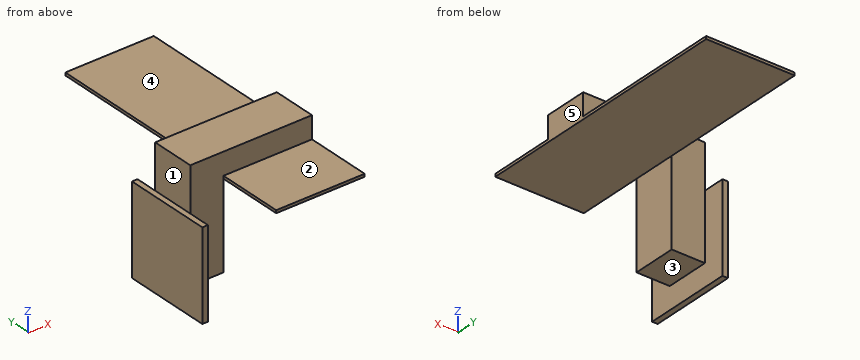
from build123d import *

# Parameters (mm, degrees)
F0_W     = 101.6
F0_H     = 304.8
F1_DEPTH = 3.175
F2_W     = 38.1
F2_H     = 50.8
F2_W_2   = 101.6
F3_DEPTH = 25.4
F4_DEPTH = 101.6
F6_DEPTH = 6.35


# Not quite as in the source:
# - the program builds the solid bodies; features that only make, move or delete a surface that nothing else refers to are left out


with BuildPart() as f1:
    # F0 (on Top) → F1 (new body)
    with BuildSketch(Plane.XY):
        with Locations((17.6723517966, 8.8070686907)):
            Rectangle(F0_W, F0_H)
    extrude(amount=F1_DEPTH)

    # F2 (on face) → F3 (join)
    with BuildSketch(Plane.XY.offset(3.175)):
        with Locations((-52.1776482034, -41.9929313093)):
            Rectangle(F2_W, F2_H)
        with Locations((17.6723517966, -41.9929313093)):
            Rectangle(F2_W_2, F2_H)
    extrude(amount=F3_DEPTH)

    # F4 (add): a face of the model
    f4_faces = [f1.faces().sort_by_distance(p)[0] for p in [
        (-52.1776482034, -41.9929313093, 3.175),
    ]]
    extrude(f4_faces, amount=F4_DEPTH)

    # F5 (on face) → F6 (join)
    with BuildSketch(Plane(origin=(-71.2276482034, 0, 0), x_dir=(0, -1, 0), z_dir=(-1, 0, 0))):
        Polygon((92.7929313093, -123.825), (92.7929313093, -22.225), (67.3929313093, -22.225), (67.3929313093, -98.425), (41.9929313093, -98.425), (16.5929313093, -98.425), (16.5929313093, -22.225), (-8.8070686907, -22.225), (-8.8070686907, -123.825), align=None)
        Polygon((67.3929313093, -98.425), (67.3929313093, -22.225), (16.5929313093, -22.225), (16.5929313093, -98.425), (41.9929313093, -98.425), align=None)
    extrude(amount=F6_DEPTH)


solid = f1.part
Geometry: final body of the model. Coordinates: model frame, mm. Face numbers are marked on the shaded views. A direction names the side the tool comes from. Give positions to 0.01 mm unless a question says otherwise; leave off trailing zeros. Loops run counter-clockwise (first coordinate to the right, second up) from the corner with the lowest first, then second, coordinate; pieces in that order, holes last. Notation, with made-up numbers: (6.5, 86) -> (52.5, 86) arc R34 cw to (52.5, 118) -> close; hole circle Ø1 at (59.25, -17.75). An arc over 180 degrees is marked (long way). Put each result on its own line as item: value.
1. Cut plane A-A (y = -84). Return the cut outline in (x, z) (3 decimals), plus the area to 3 significant figures.
Taken from the geometry:
outline: (-77.578, -123.825) -> (-71.228, -123.825) -> (-71.228, -22.225) -> (-77.578, -22.225) -> close; (-33.128, 0) -> (68.472, 0) -> (68.472, 3.175) -> (-33.128, 3.175) -> close
area: 968 mm2
2. Cut plane D-D (y = -32.5). Return the cut outline in (x, z) (3 decimals).
Taken from the geometry:
outline: (-77.578, -123.825) -> (-71.228, -123.825) -> (-71.228, -98.425) -> (-33.128, -98.425) -> (-33.128, 0) -> (68.472, 0) -> (68.472, 28.575) -> (-71.228, 28.575) -> (-71.228, -22.225) -> (-77.578, -22.225) -> close
3. Pin query (flat end, axial travel): P1, Ø1.6, axis at y = 97.5, z = 2, coming from the -X side; P2, Ø11.5, axis at x = -53.5, y = -50, coming from the -Z side (3 decimals); P3, Ø2, axis at x = 46, y = -104, coming from the -Z side. Return the tip coordinate at first contact, or that it passes through.
Taken from the geometry:
P1: stops at x = -33.13
P2: stops at z = -98.425
P3: stops at z = 0
4. Ray query, line 1 along Z through (x, y) = (-22, -116.5) (3 decimals); line 2 along X through (y, z) = (-23.5, -114.5); line 3 along X through (y, z) = (-57.5, -22). Return the intervals inside material, ascending. Write a range as [from, to].
Taken from the geometry:
line 1: z = [0, 3.175]
line 2: x = [-77.58, -71.23]
line 3: x = [-71.23, -33.13]
5. Set-up query: the marked faces 1, 2, 3, 4 and 5. Return all of +Z, -Z, +X, -X, +Y, -Y with unobstructed straight access to the full face (end or side cutting, diameter ignored); none if empty.
Taken from the geometry:
face 1: +Z, -X, +Y, -Y
face 2: +Z, +X, -X, -Y
face 3: -Z, +X, +Y, -Y
face 4: +Z, +X, -X, +Y
face 5: +Z, -Z, +X, +Y, -Y
6. Cut plane C-C (x = 44). Return the cut outline in (y, z) (3 decimals).
Taken from the geometry:
outline: (-143.593, 0) -> (161.207, 0) -> (161.207, 3.175) -> (-16.593, 3.175) -> (-16.593, 28.575) -> (-67.393, 28.575) -> (-67.393, 3.175) -> (-143.593, 3.175) -> close
7. Cut plane B-B (z = -94). Return the cut outline in (x, y), plus the area to 3 significant figures.
Taken from the geometry:
outline: (-77.58, -92.79) -> (-71.23, -92.79) -> (-71.23, -67.39) -> (-33.13, -67.39) -> (-33.13, -16.59) -> (-71.23, -16.59) -> (-71.23, 8.81) -> (-77.58, 8.81) -> close
area: 2,580 mm2
